For this review, use the dimensioned drawing (mm, ordinates from the lowest corner) and the shaded views. A direction names the side the tool comes from. Round coordinates to 2 decimals unless told otherwise and drop trailing zeros. Loops run counter-clockwise (first coordinate to the right, second up) from the corner with the lowest first, then second, coordinate; pieces in that order, holes last. Notation, with made-up numbers: (17.25, 33) - (46.25, 33) arc R22 cw to (46.25, 69) - close; hole circle Ø9 at (38.25, 27). An arc over 180 degrees is marked (long way). Answer as CSV lines item,"result". Start each with the question number.
(1) For P1, Ø3, axis at x = 75, z = 186, coming from the +Y side; P2, Ø15, axis at y = 127, z = 195.5, coming from the -X side (3 decimals); P3, Ø9.5, axis at y = 123, z = 32, coming from the +X side (3 decimals), all flat-tipped, find the tip position at first contact; note any pin that passes through.
(2) Consider section B-B (y = 67.5). Give the boundary of the cut face in (x, z).
(3) Wall thickness on L1, parallel to Y at x = 32, z = 118.5; L2, parallel to X at y = 115, z = 25 (3 decimals); L3, parallel to Y at x = 79, z = 53.5: over which ranges is each line inside the solid? List them lowest first.
(4) Consider section C-C (z = 115). Give the boundary of the cut face in (x, y).
(5) For the marked faces 1, 2, 3 and 4, list the 3-axis set-ups (+Z, -Z, +X, -X, +Y, -Y) from which the entire face can be reached by the end or side of a thin tool; tool diameter is ignored.
(6) Consider section A-A (x = 118.5). Give the boundary of the cut face in (y, z).
(7) Consider section D-D (y = 9). Give the boundary of the cut face in (x, z), and give its area (3 significant figures).
(8) Mouldability with a two-part tool opening along Y and no side actions: class the marked faces 5, 6, 7 and 8 as released by +Y, released by -Y, zero draft, split by the parting line, or undercut.
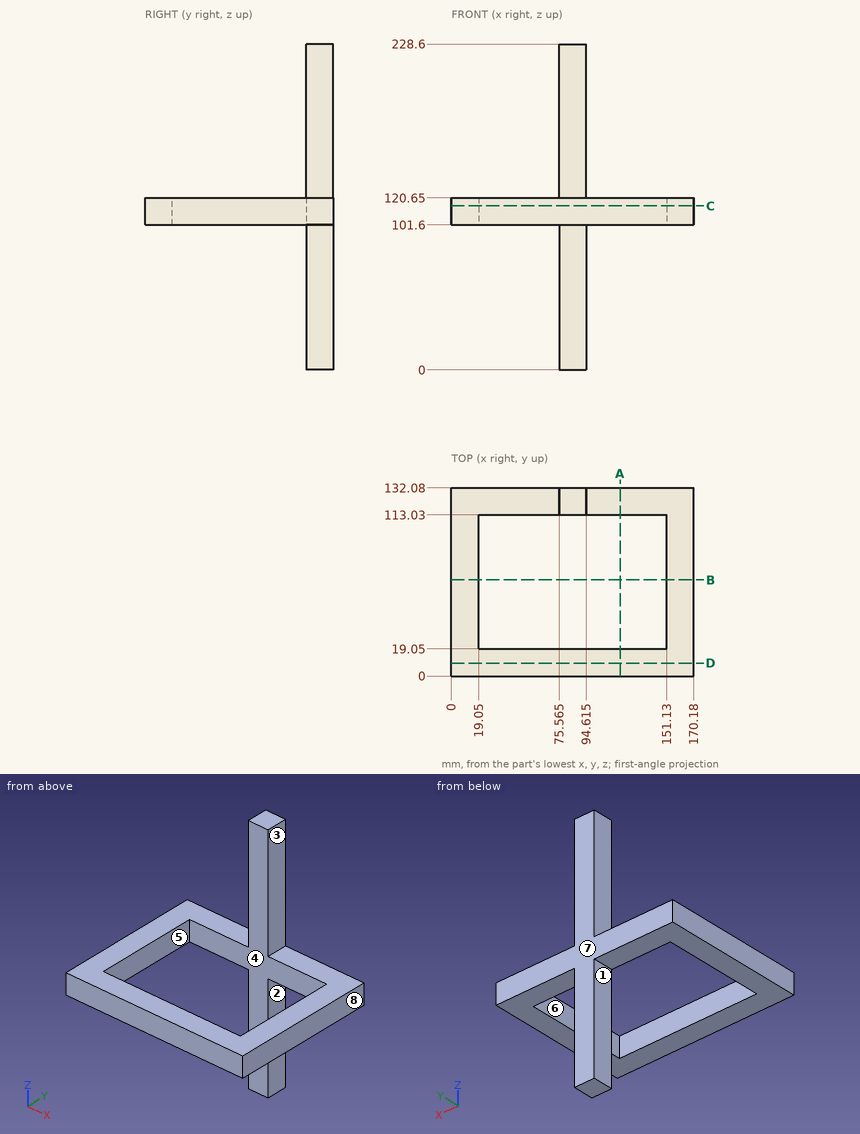
Determined:
1,P1,"stops at y = 132.08"
1,P2,"stops at x = 75.565"
1,P3,"stops at x = 94.615"
2,outline,"(0, 101.6) - (19.05, 101.6) - (19.05, 120.65) - (0, 120.65) - close; (151.13, 101.6) - (170.18, 101.6) - (170.18, 120.65) - (151.13, 120.65) - close"
3,L1,"y = 0 to 19.05, 113.03 to 132.08"
3,L2,"x = 75.565 to 94.615"
3,L3,"y = 113.03 to 132.08"
4,outline,"(0, 0) - (170.18, 0) - (170.18, 132.08) - (0, 132.08) - close; hole (19.05, 19.05) - (151.13, 19.05) - (151.13, 113.03) - (19.05, 113.03) - close"
5,face 1,"-Z, -X, +Y, -Y"
5,face 2,"-Z, +X, +Y, -Y"
5,face 3,"+Z, +X, +Y, -Y"
5,face 4,"+Z, -Z"
6,outline,"(0, 101.6) - (19.05, 101.6) - (19.05, 120.65) - (0, 120.65) - close; (113.03, 101.6) - (132.08, 101.6) - (132.08, 120.65) - (113.03, 120.65) - close"
7,outline,"(0, 101.6) - (170.18, 101.6) - (170.18, 120.65) - (0, 120.65) - close"
7,area,"3,240 mm^2"
8,face 5,"undercut"
8,face 6,"undercut"
8,face 7,"released by +Y"
8,face 8,"zero draft"
